Study the drawing (mm; zero at the part's minimum x, y, z) and answer. Coordinates: 2 decimals unless noted, no trailing zeros. Order: outer loops, then holes, each group sorted by start corner. A loop starts at its lowest first (then second) coordinate and runs counter-clockwise, first axis right, second up. Notation, with made-up numbers: M 83,51.5 L 131,51.5 A26 cw 131,66.5 Z; hole C -30.5,-8 d10. An arc over 180 degrees is marked long. Put each result on its own line as item: value.
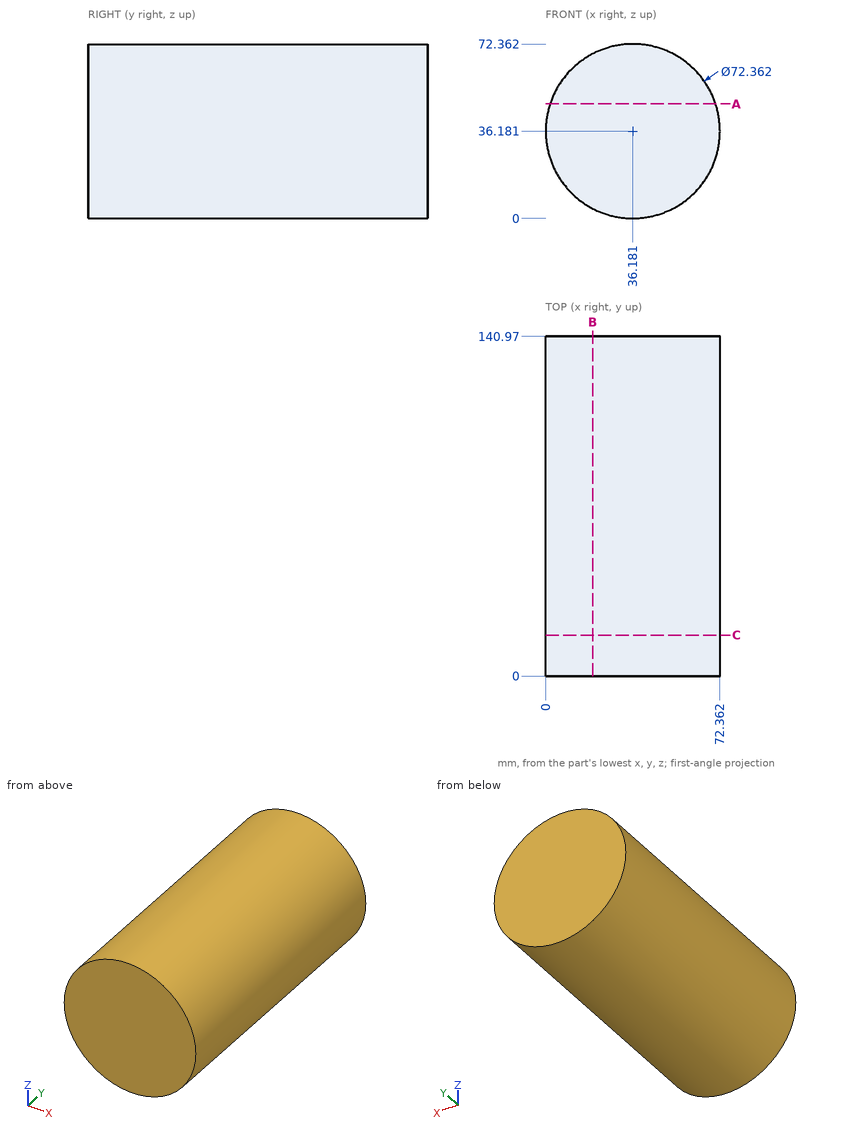
Q1. Find section B-B on x = 19.5. Write down the section's boundary in (y, z) (1 decimal), plus the area to 3 significant figures.
Answers below:
outline: M 0,4.1 L 141,4.1 L 141,68.3 L 0,68.3 Z
area: 9,050 mm^2
Q2. Find section C-C on y = 17. Write down the section's boundary in (x, z).
Answers below:
outline: C 36.18,36.18 d72.36
Q3. Given pin 1 (1 mm diameter, centred on y = 123.5, z = 28, fed in from +X); pin 2 (5 mm diameter, centred on y = 50.5, z = 27.5, fed in from +X); pin 3 (10 mm diameter, centred on y = 102.5, z = 58.5, fed in from +X), each flat-ended and moving along its own axis, determine where each tip first touches the part or whether it passes through.
Answers below:
pin 1: stops at x = 71.54
pin 2: stops at x = 71.83
pin 3: stops at x = 67.95
Q4. Consider line 1 along X through (y, z) = (17, 36.5); line 2 along X through (y, z) = (16, 35); line 3 along Z through (x, y) = (20, 116). Determine where each line is inside the solid, lowest interval first.
Answers below:
line 1: x = 0 to 72.36
line 2: x = 0.02 to 72.34
line 3: z = 3.82 to 68.54
Q5. Find section A-A on z = 47.5. Write down the section's boundary in (x, y), plus the area to 3 significant figures.
Answers below:
outline: M 1.82,0 L 70.55,0 L 70.55,140.97 L 1.82,140.97 Z
area: 9,690 mm^2
